Part model, mm, in its own coordinate system. A direction names the side the tool comes from. Coordinates: 2 decimals unless noted, no trailing zeros. Use a Markdown table: item, result. Add a question column.
Q1. Slice it at A-A on z = 0. Count the separate pieces of the cut face and the enclosed holes in it, then the cut area to 3 significant figures.
Q2. Mould opens along Z. For faces 1 (the conical face through (3.216, -21.465, -13.536)), 2 (the flat face through (0, -13.878, -11)), 3 (the conical face through (2.4, -17.25, -10.11)), 4 (the flat face through (-4.856, -18.668, 12.018)) say: released by +Z, released by -Z, zero draft, split by the parting line, or undercut.
Q3. Pin check, flat tips, straight feed: pin 1 Ø9.5 at (x, z) = (-2.5, 4.5) entering from -Y; pin 2 Ø17 at (x, z) = (4.5, 0.5) entering from -Y; pin 3 Ø1 at (y, z) = (-16, 4) entering from -X. Stop position of each tip, or through.
Q4. Tool access for faces 5 (the flat face through (7.2, -21.628, -8.2)), 6 (the conical face through (2.4, -16.53, -10.11)), 7 (the flat face through (0, -19, 13)): list every direction of +Z, -Z, +X, -X, +Y, -Y with a clear straight run to the whole face (end or side of a thin tool).
Q5. Wall check: L1, parallel to X at y = -18.6, z = 0; L2, parallel to X at y = -17.25, z = 1.5; L3, parallel to X at y = -18, z = 13. Give the ranges that are in metal, low to high. Write a range as from..to.
from build123d import *

# Parameters (mm, degrees)
F2_ANGLE = 338
F3_R     = 29.1
F3_R_2   = 17.1
F4_DEPTH = 25


with BuildPart() as f2:
    # F1 (on Right) → F2 (revolve)
    with BuildSketch(Plane.YZ):
        Polygon((-14.592193, 10.25), (-13.878119, 10.75), (-13.878119, 20.5), (-14.878119, 20.5), (-21.628119, 13.75), (-21.628119, 10.75), (-17.448489, 10.75), (-17.448489, 10.25), (-16.734415, 10.75), (-16.734415, 10.25), (-16.020341, 10.75), (-16.020341, 10.25), (-15.306267, 10.75), (-15.306267, 10.25), (-14.592193, 10.75), align=None)
    revolve(axis=Axis((0, -8.217514, 0), (0, 1, 0)), revolution_arc=F2_ANGLE)

    # F3 (on Front) → F4 (cut)
    with BuildSketch(Plane.XZ):
        Circle(F3_R)
        Circle(F3_R_2, mode=Mode.SUBTRACT)
    extrude(amount=F4_DEPTH, mode=Mode.SUBTRACT)

    # F5 (on face) → F6 (revolve, cut)
    with BuildSketch(Plane(origin=(0, 0, 0), x_dir=(0, 1, 0), z_dir=(0.927184, 0, 0.374607))):
        Polygon((-15.378119, 11.75), (-15.378119, 15.6), (-17.656798, 15.6), (-19.254081, 14.002717), (-17.001364, 11.75), align=None)
    revolve(axis=Axis((0, -8.217514, 0), (0, 1, 0)), mode=Mode.SUBTRACT)


solid = f2.part
Recorded:
| question | item | result |
|---|---|---|
| 1 | separate pieces | 2 |
| 1 | enclosed holes | 2 |
| 1 | area | 66.8 mm² |
| 2 | face 1 | split by the parting line |
| 2 | face 2 | zero draft |
| 2 | face 3 | undercut |
| 2 | face 4 | released by +Z |
| 3 | pin 1 | through |
| 3 | pin 2 | y = -21.63 |
| 3 | pin 3 | x = -16.74 |
| 4 | face 5 | +Z, -Z, +X, -X, -Y |
| 4 | face 6 | none |
| 4 | face 7 | +Z, +Y, -Y |
| 5 | L1 | -16.78..-14.66, -13.35..-10.75, 10.75..13.35, 14.66..16.78 |
| 5 | L2 | -17.03..-15.53, -11.9..-10.28, 10.28..11.9, 15.53..17.03 |
| 5 | L3 | -11.11..-7.99, 7.99..11.11 |
